Autodesk Inventor part; units mm, degrees
ref_plane "YZ Plane" through (0, 0, 0) normal (1, 0, 0) x (0, 1, 0)
ref_plane "XZ Plane" through (0, 0, 0) normal (0, 1, 0) x (-1, 0, 0)
ref_plane "XY Plane" through (0, 0, 0) normal (0, 0, 1) x (1, 0, 0)
sketch "Sketch1" plane through (0, 0, 0) normal (0, 0, 1) x (1, 0, 0)
  line L0 (0, 0) -> (96, 0)
  line L1 (96, 0) -> (96, 80)
  line L2 (96, 80) -> (0, 80)
  line L3 (0, 80) -> (0, 0)
  dimension "d0" = 96
  dimension "d1" = 80
extrude "Extrusion1" add sketch "Sketch1" along normal blind 13
sketch "Sketch2" plane through (0, 80, 0) normal (0, 1, 0) x (1, 0, 0)
  line L0 (3, -13) -> (93, -13)
  line L1 (93, -13) -> (93, -3)
  line L2 (93, -3) -> (3, -3)
  line L3 (3, -3) -> (3, -13)
  line L4 (0, 0) -> (0, -13)
  line L5 (96, 0) -> (0, 0)
  line L6 (96, 0) -> (96, -13)
  dimension "d4" = 3
  dimension "d5" = 3
  dimension "d6" = 3
extrude "Extrusion2" cut sketch "Sketch2" against normal through all
sketch "Sketch3" plane through (96, 0, 0) normal (1, 0, 0) x (0, 0, -1)
  line L0 (0, 80) -> (-13, 80) construction
  line L1 (-6.5, 80) -> (-6.5, 0) construction
  line L2 (0, 0) -> (-13, 0) construction
  line L3 (-13, 0) -> (-13, 80) construction
  line L4 (0, 0) -> (0, 80)
  point P0 (-6.5, 75)
  point P1 (-6.5, 5)
  dimension "d17" = 70
  dimension "d18" = 5
  dimension "d19" = 6.5
hole "Hole1" at (96, 75, 6.5) at (96, 5, 6.5) direction (-1, 0, 0) diameter 3 end through all
properties part number "Mirror_shell_adapter"
Input: part model. Units: mm. Frame: model coordinates. A direction names the side the tool comes from. Coordinates: 2 decimals unless noted, no trailing zeros. Write each loop counter-clockwise with the first axis right and the second up, starting at its lowest first coordinate (ties: lowest second). Pieces come first, ordered by that corner, then holes. Notation, with made-up numbers: M -33,75.5 L -7,75.5 A14 cw -7,99.5 Z; hole C 70,9.5 d3. An arc over 180 degrees is marked long. Answer as a JSON object with one key per item and string values. Group by question number.
(1) Section B-B on z = 10.75. Output: boundary loops of the cut face in (x, y).
(2) Section C-C on y = 59. Output: boundary loops of the cut face in (x, z).
(3) Ray query, line 1 along Y through (x, z) = (94.55, 6.5); line 2 along X through (y, z) = (72.5, 9.75); line 3 along Z through (x, y) = (94, 5). Return the intervals inside material, ascending. Write a range as [from, to].
(4) Mould query, pull axis Y, two halves, no side actions, for faces 3 (the face through (1.48, 3.99, 7.61)), 4 (the face through (96, 39, 6)), 5 (the face through (48, 0, 2)). Classes: pulls with the +Y half, pulls with the -Y half, needs draft (parallel to the pull), parting line crosses it, or undercut.
(5) Set-up query: faces 1 (the face through (1, 41, 13)), 2 (the face through (93, 41, 8)). Return all of +Z, -Z, +X, -X, +Y, -Y with unobstructed straight access to the full face (end or side cutting, diameter ignored); none if empty.
(6) Section D-D on x = 49.5. Output: boundary loops of the cut face in (y, z), plus the area to 3 significant figures.
(7) Section A-A on y = 75. Output: boundary loops of the cut face in (x, z), plus the area to 3 significant figures.
Result set:
{
 "1": {"outline": "M 0,0 L 3,0 L 3,80 L 0,80 Z; M 93,0 L 96,0 L 96,80 L 93,80 Z"},
 "2": {"outline": "M 0,0 L 96,0 L 96,13 L 93,13 L 93,3 L 3,3 L 3,13 L 0,13 Z"},
 "3": {"line 1": "y = [0, 3.5], [6.5, 73.5], [76.5, 80]", "line 2": "x = [0, 3], [93, 96]", "line 3": "z = [0, 5], [8, 13]"},
 "4": {"face 3": "undercut", "face 4": "needs draft", "face 5": "pulls with the -Y half"},
 "5": {"face 1": "+Z, +X, -X, +Y, -Y", "face 2": "+Z, +Y, -Y"},
 "6": {"outline": "M 0,0 L 80,0 L 80,3 L 0,3 Z", "area": "240 mm2"},
 "7": {"outline": "M 0,0 L 96,0 L 96,5 L 93,5 L 93,3 L 3,3 L 3,5 L 0,5 Z; M 0,8 L 3,8 L 3,13 L 0,13 Z; M 93,8 L 96,8 L 96,13 L 93,13 Z", "area": "330 mm2"}
}
